The listing builds one solid part. Answer for the finished solid, in the listing's coordinates (mm). Face numbers are marked on the shaded views. A direction names the side the tool comes from. Coordinates: 2 decimals unless noted, no trailing zeros. Order: outer loops, then holes, each group sorted by start corner. A loop starts at its lowest first (then second) coordinate and runs counter-clockwise, first axis right, second up. Notation, with made-up numbers: (41, 44.5) -> (97, 44.5) arc R14 ccw to (97, 49.5) -> close; hole circle Ø3 at (38.25, 67). An arc over 180 degrees is marked (long way). Return JSON: item names as keys, results as strings.
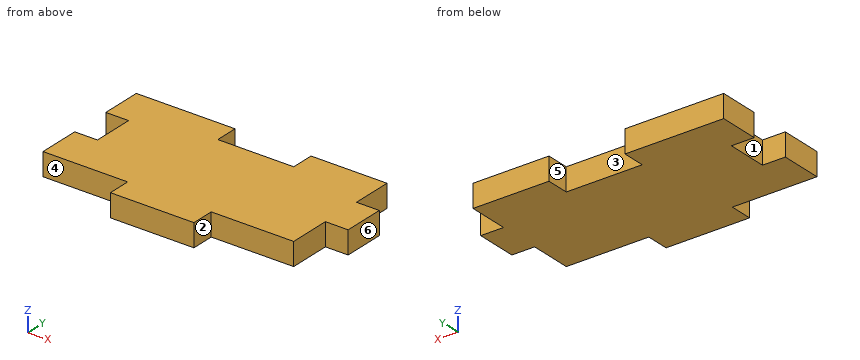
from build123d import *

# Parameters (mm, degrees)
BOSS_EXTRUDE1_DEPTH = 5
CAVITY1_START       = 8.5
CAVITY1_OUTLINE_W   = 16.666666666
CAVITY1_OUTLINE_H   = 5
CAVITY1_DEPTH       = 5


# Read off the part's stored shape, not the designer's step: Cavity1
with BuildPart() as part:
    # Sketch1 → Boss-Extrude1 (new body)
    with BuildSketch(Plane.XY):
        Polygon((27.5, 4.666666667), (27.5, 13.5), (-27.5, 13.5), (-27.5, 4.666666667), (-22.5, 4.666666667), (-22.5, -4.333333333), (-27.5, -4.333333333), (-27.5, -13.5), (-8.924137908, -13.5), (-8.924137908, -18.5), (9.409195426, -18.5), (9.409195426, -13.5), (27.5, -13.5), (27.5, -4.333333333), (32.5, -4.333333333), (32.5, 4.666666667), align=None)
    extrude(amount=BOSS_EXTRUDE1_DEPTH)

    # Cavity1 outline → Cavity1 (cut)
    with BuildSketch(Plane(origin=(0, 0, 0), x_dir=(1, 0, 0), z_dir=(0, 1, 0)).offset(CAVITY1_START)):
        with Locations((2.5, -2.5)):
            Rectangle(CAVITY1_OUTLINE_W, CAVITY1_OUTLINE_H)
    extrude(amount=CAVITY1_DEPTH, mode=Mode.SUBTRACT)


solid = part.part
1. For the marked faces 1, 2 and 3, determine the directions among +Z, -Z, +X, -X, +Y, -Y from which every point of the face is accessible in a straight line to the end or side of a thin tool.
Answer block:
{"face 1": "+Z, -Z, -X", "face 2": "+Z, -Z, +X, -Y", "face 3": "+Z, -Z, +Y"}
2. The part is cut by section A-A on y = 12. Give the vertices of the cut face in (x, z).
Answer block:
{"outline": "(-27.5, 0) -> (-5.83, 0) -> (-5.83, 5) -> (-27.5, 5) -> close; (10.83, 0) -> (27.5, 0) -> (27.5, 5) -> (10.83, 5) -> close"}
3. Each of these flat-tipped pins is pushed along its axis until it touches: pin 1 Ø2.5 at (x, z) = (30.5, 3.5) entering from -Y; pin 2 Ø2 at (y, z) = (-11, 1.5) entering from +X; pin 3 Ø1.5 at (x, y) = (2.5, 0) entering from -Z; pin 4 Ø1.5 at (x, z) = (16.5, 3.5) entering from -Y. Where does it stop, or does it pass through?
Answer block:
{"pin 1": "stops at y = -4.33", "pin 2": "stops at x = 27.5", "pin 3": "stops at z = 0", "pin 4": "stops at y = -13.5"}
4. The part is cut by section B-B on z = 2. Give the vertices of the cut face in (x, y), and give its area (3 significant figures).
Answer block:
{"outline": "(-27.5, -13.5) -> (-8.92, -13.5) -> (-8.92, -18.5) -> (9.41, -18.5) -> (9.41, -13.5) -> (27.5, -13.5) -> (27.5, -4.33) -> (32.5, -4.33) -> (32.5, 4.67) -> (27.5, 4.67) -> (27.5, 13.5) -> (10.83, 13.5) -> (10.83, 8.5) -> (-5.83, 8.5) -> (-5.83, 13.5) -> (-27.5, 13.5) -> (-27.5, 4.67) -> (-22.5, 4.67) -> (-22.5, -4.33) -> (-27.5, -4.33) -> close", "area": "1,490 mm2"}
5. Consider line 1 (Y direction, x = 12.5, z = 3.25); line 2 (Y direction, x = -25, z = 1.6); line 3 (X direction, y = 4.5, z = 1.1). Determine where each line is inside the solid, lowest interval first. Write a range as from..to.
Answer block:
{"line 1": "y = -13.5..13.5", "line 2": "y = -13.5..-4.33, 4.67..13.5", "line 3": "x = -22.5..32.5"}
6. Determine the mould class of the marked faces 4, 5 and 6 for opening direction X: pulls with the +X half, pulls with the -X half, needs draft (parallel to the pull), parting line crosses it, or undercut.
Answer block:
{"face 4": "needs draft", "face 5": "undercut", "face 6": "pulls with the +X half"}
7. The part is cut by section C-C on x = -15. Give the vertices of the cut face in (y, z), and give its area (3 significant figures).
Answer block:
{"outline": "(-13.5, 0) -> (13.5, 0) -> (13.5, 5) -> (-13.5, 5) -> close", "area": "135 mm2"}
8. The part is cut by section D-D on y = -9. Give the vertices of the cut face in (x, z), and give its area (3 significant figures).
Answer block:
{"outline": "(-27.5, 0) -> (27.5, 0) -> (27.5, 5) -> (-27.5, 5) -> close", "area": "275 mm2"}
